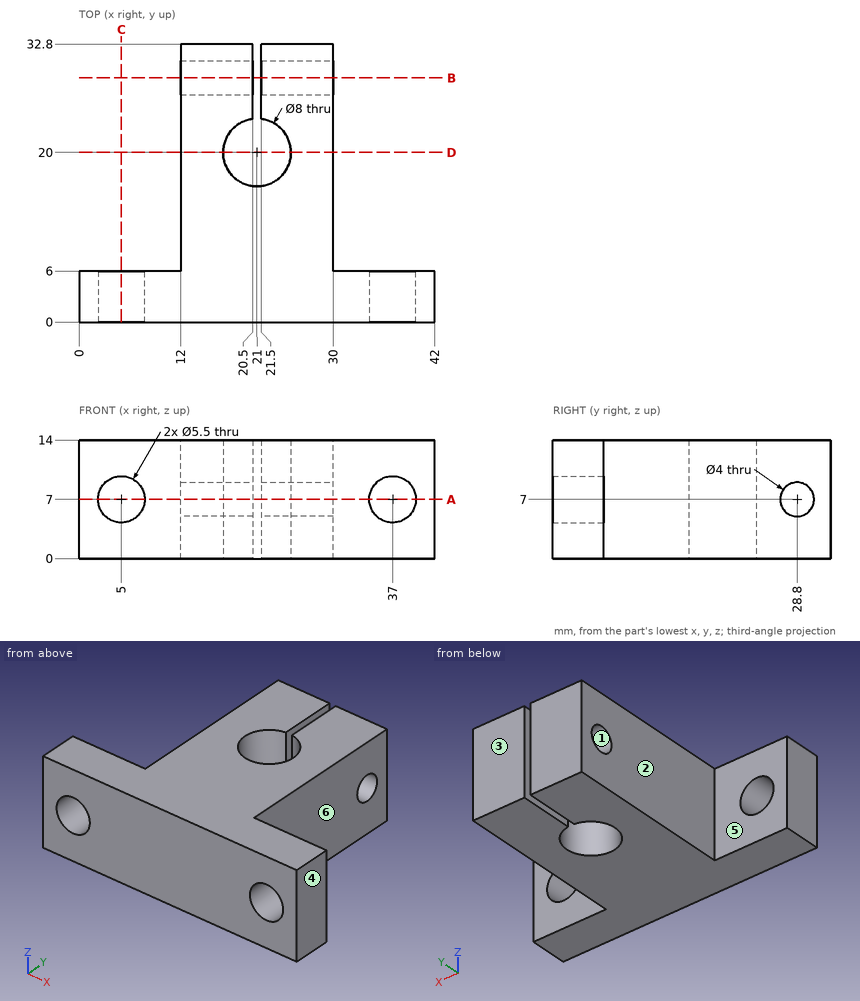
Check sheet for the drawn part. Datum: minimum x, y, z corner. Units: mm. A direction names the side the tool comes from. Round coordinates to 2 decimals unless told otherwise and drop trailing zeros. Write each loop counter-clockwise with the first axis right and the second up, starting at its lowest first coordinate (ties: lowest second). Pieces come first, ordered by that corner, then holes. Notation, with made-up numbers: (-22, -39) -> (-18, -39) arc R19 ccw to (-18, -16) -> close; hole circle Ø3 at (66.5, 26.25). An arc over 180 degrees is marked (long way). Write each question's results on one line, items separated by ' | '.
Q1. Sectioned sample at B-B, the plane y = 28.8. Record the boundary of the cut face in (x, z).
Derived:
outline: (12, 0) -> (20.5, 0) -> (20.5, 5) -> (12, 5) -> close; (12, 9) -> (20.5, 9) -> (20.5, 14) -> (12, 14) -> close; (21.5, 0) -> (30, 0) -> (30, 5) -> (21.5, 5) -> close; (21.5, 9) -> (30, 9) -> (30, 14) -> (21.5, 14) -> close
Q2. Thickness scan on probe 1 along X at (y, z) = (5.5, 5); probe 2 along X at (y, z) = (20, 6.75); probe 3 along X at (y, z) = (27.5, 2.5). Record the ranges inside material, lowest first.
Derived:
probe 1: x = 0 to 3.11, 6.89 to 35.11, 38.89 to 42 | probe 2: x = 12 to 17, 25 to 30 | probe 3: x = 12 to 20.5, 21.5 to 30
Q3. Draft check along Y on the marked faces 1, 2 and 3. Enter one of: released by +Y, released by -Y, zero draft, split by the parting line, or undercut.
Derived:
face 1: undercut | face 2: zero draft | face 3: released by +Y
Q4. Sectioned sample at A-A, the plane z = 7. Record the boundary of the cut face in (x, y).
Derived:
outline: (0, 0) -> (2.25, 0) -> (2.25, 6) -> (0, 6) -> close; (7.75, 0) -> (34.25, 0) -> (34.25, 6) -> (30, 6) -> (30, 26.8) -> (21.5, 26.8) -> (21.5, 23.97) arc R4 cw (long way) to (20.5, 23.97) -> (20.5, 26.8) -> (12, 26.8) -> (12, 6) -> (7.75, 6) -> close; (12, 30.8) -> (20.5, 30.8) -> (20.5, 32.8) -> (12, 32.8) -> close; (21.5, 30.8) -> (30, 30.8) -> (30, 32.8) -> (21.5, 32.8) -> close; (39.75, 0) -> (42, 0) -> (42, 6) -> (39.75, 6) -> close
Q5. Sectioned sample at C-C, the plane x = 5. Record the boundary of the cut face in (y, z), and give its area (3 significant figures).
Derived:
outline: (0, 0) -> (6, 0) -> (6, 4.25) -> (0, 4.25) -> close; (0, 9.75) -> (6, 9.75) -> (6, 14) -> (0, 14) -> close | area: 51.0 mm²
Q6. Access from +Z, -Z, +X, -X, +Y, -Y to the whole of each face (thin tool, end or side, straight path). Record for the marked faces 4, 5 and 6.
Derived:
face 4: +Z, -Z, +X, +Y, -Y | face 5: +Z, -Z, -X, +Y | face 6: +Z, -Z, +X, +Y
Q7. Sectioned sample at D-D, the plane y = 20. Record the boundary of the cut face in (x, z), and give its area (3 significant figures).
Derived:
outline: (12, 0) -> (17, 0) -> (17, 14) -> (12, 14) -> close; (25, 0) -> (30, 0) -> (30, 14) -> (25, 14) -> close | area: 140 mm²
Q8. Go/stop test with flat-tipped pins: pin 1 Ø4 at (y, z) = (12, 10.5) entering from -X; pin 2 Ø4.5 at (y, z) = (28.8, 7) entering from +X; pin 3 Ø6 at (x, z) = (6, 10) entering from +Y. Record where each tip stops, or that it passes through.
Derived:
pin 1: stops at x = 12 | pin 2: stops at x = 30 | pin 3: stops at y = 6
